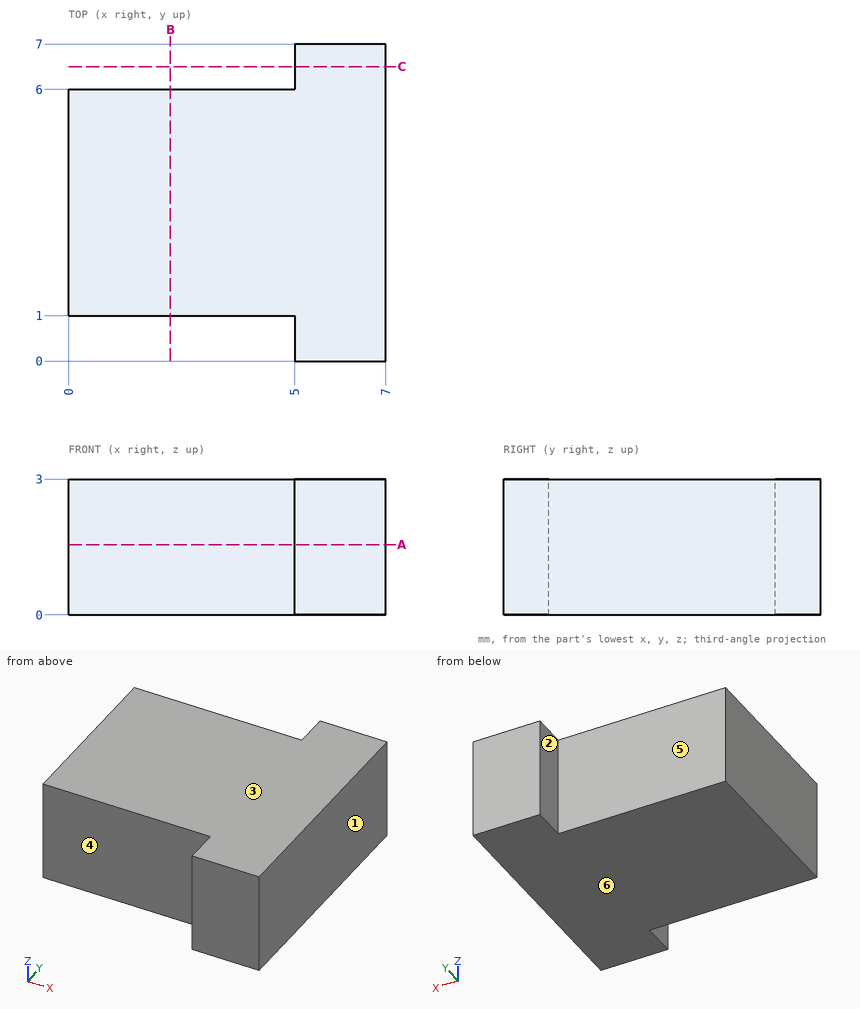
Input: dimensioned drawing with shaded views. Units: mm. Origin: part minimum x, y, z. A direction names the side the tool comes from. Round coordinates to 2 decimals unless told otherwise and drop trailing zeros. Order: outer loops, then holes, each group sorted by start corner. A loop starts at its lowest first (then second) coordinate and runs counter-clockwise, first axis right, second up.
Q1. Section B-B, the plane x = 2.25. Output: boundary loops of the cut face in (y, z).
Result sheet:
outline: (1, 0) - (6, 0) - (6, 3) - (1, 3) - close
Q2. Section C-C, the plane y = 6.5. Output: boundary loops of the cut face in (x, z), and give its area (3 significant figures).
Result sheet:
outline: (5, 0) - (7, 0) - (7, 3) - (5, 3) - close
area: 6.00 mm2
Q3. Pin query (flat end, axial travel): pin 1 (0.9 mm diameter, centred on x = 3, z = 1.5, fed in from -Y); pin 2 (0.5 mm diameter, centred on y = 0.5, z = 1.5, fed in from -X); pin 3 (0.9 mm diameter, centred on x = 3.5, z = 2, fed in from +Y). Return the tip coordinate at first contact, or that it passes through.
Result sheet:
pin 1: stops at y = 1
pin 2: stops at x = 5
pin 3: stops at y = 6
Q4. Mould query, pull axis X, two halves, no side actions, for the marked faces 1, 2 and 3. Classes: released by +X, released by -X, zero draft, split by the parting line, or undercut.
Result sheet:
face 1: released by +X
face 2: released by -X
face 3: zero draft
Q5. Material intervals for probe 1 along Y at (x, z) = (0.5, 2.75); probe 2 along X at (y, z) = (6.5, 1.4), sorted ascending.
Result sheet:
probe 1: y = 1 to 6
probe 2: x = 5 to 7
Q6. Access query for the marked faces 4, 5 and 6. Directions: +Z, -Z, +X, -X, +Y, -Y. A direction counts if a zero-diameter tool reaches every point of the face in a straight line with its end or side. Return the directions, or none.
Result sheet:
face 4: +Z, -Z, -X, -Y
face 5: +Z, -Z, -X, +Y
face 6: -Z, +X, -X, +Y, -Y
Q7. Section A-A, the plane z = 1.55. Output: boundary loops of the cut face in (x, y).
Result sheet:
outline: (0, 1) - (5, 1) - (5, 0) - (7, 0) - (7, 7) - (5, 7) - (5, 6) - (0, 6) - close
